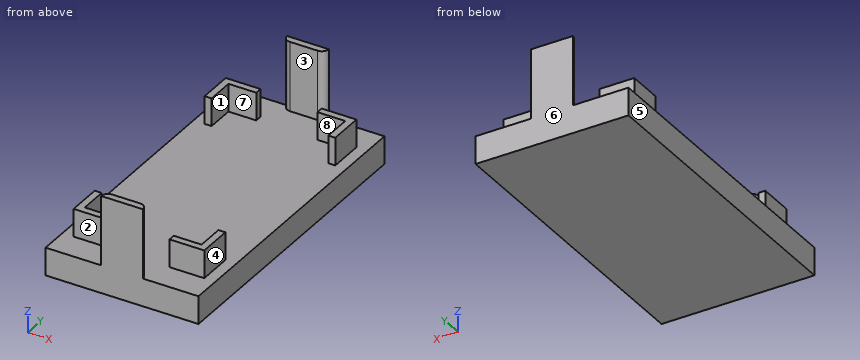
```python
from build123d import *

# Parameters (mm, degrees)
F0_W     = 110
F0_H     = 220
F1_DEPTH = 20
F3_DEPTH = 20
F4_W     = 30
F4_H     = 5
F5_DEPTH = 50
F6_R     = 4.99999


# Not quite as in the source:
# - a fillet or chamfer is up to 0.001 mm smaller than in the source, because OpenCascade refuses the exact size


with BuildPart() as f1:
    # F0 (on Top) → F1 (new body)
    with BuildSketch(Plane.XY):
        with Locations((55, -110)):
            Rectangle(F0_W, F0_H)
    extrude(amount=F1_DEPTH)

    # F2 (on face) → F3 (join)
    with BuildSketch(Plane.XY.offset(20)):
        Polygon((8, -20), (8, -45), (13, -45), (13, -25), (33, -25), (33, -20), align=None)
        Polygon((77, -20), (77, -25), (97, -25), (97, -45), (102, -45), (102, -20), align=None)
        Polygon((33, -200), (33, -195), (13, -195), (13, -175), (8, -175), (8, -200), align=None)
        Polygon((97, -175), (97, -195), (77, -195), (77, -200), (102, -200), (102, -175), align=None)
    extrude(amount=F3_DEPTH)

    # F4 (on face) → F5 (join)
    with BuildSketch(Plane.XY.offset(20)):
        with Locations((55, -2.5)):
            Rectangle(F4_W, F4_H)
        with Locations((55, -217.5)):
            Rectangle(F4_W, F4_H)
    extrude(amount=F5_DEPTH)

    # F6 (radius 5 in the source; OpenCascade refuses exactly that, so slightly less here)
    f6_edges = [f1.edges().sort_by_distance(p)[0] for p in [
        (40, -5, 45),
        (70, -5, 45),
        (40, -215, 45),
        (70, -215, 45),
    ]]
    fillet(f6_edges, radius=F6_R)


solid = f1.part
```
Here's how the part is built. I have some questions about the finished solid (model axes, mm). Face numbers are marked on the shaded views. A direction names the side the tool comes from. Round coordinates to 2 decimals unless told otherwise and drop trailing zeros. Write each loop counter-clockwise with the first axis right and the second up, starting at its lowest first coordinate (ties: lowest second). Pieces come first, ordered by that corner, then holes. Notation, with made-up numbers: M 47.5,55 L 82.5,55 A6 cw 82.5,63 Z; hole C 27,32.25 d2. An arc over 180 degrees is marked long. Answer as CSV lines item,"result". Start each with the question number.
1. Suppose I cut it at D-D on y = -141.5. Write out the boundary of the cut face in (x, z), then the cut area to 3 significant figures.
2. I'm going to push flat-ended pins straight in: pin 1 Ø3 at (x, y) = (19, -173) entering from +Z; pin 2 Ø5.5 at (y, z) = (-196.5, 25.5) entering from -X; pin 3 Ø10 at (y, z) = (-38.5, 29) entering from +X. Where does each tip first touch, or does it pass through?
3. Suppose I cut it at C-C on z = 37. Count the separate pieces of the cut face and the enclosed holes in it, then the cut area to 3 significant figures.
4. On a 3-axis mill with a long thin cutter (end or side, diameter ignored), from which of +Z, -Z, +X, -X, +Y, -Y can I reach the whole of each face in a straight line? I mean the marked faces 1, 2, 3 and 4. Say none if no direction works.
5. Thinking about a two-plate mould opening in Y: for the marked faces 5, 6, 7 and 8, which applies, released by +Y, released by -Y, zero draft, split by the parting line, or undercut?
6. I need wall thicknesses on probe 1 along Y at (x, z) = (92, 29.5); probe 2 along Y at (x, z) = (65.5, 60); probe 3 along Z at (x, y) = (38, -16.5). Which ranges of each line are inside material? Lowest first, please.
7. Suppose I cut it at B-B on y = -41. Write out the boundary of the cut face in (x, z).
Check result:
1,outline,"M 0,0 L 110,0 L 110,20 L 0,20 Z"
1,area,"2,200 mm2"
2,pin 1,"stops at z = 20"
2,pin 2,"stops at x = 8"
2,pin 3,"stops at x = 102"
3,separate pieces,"6"
3,enclosed holes,"0"
3,area,"1,180 mm2"
4,face 1,"+Z"
4,face 2,"+Z, +X, -X, -Y"
4,face 3,"+Z, +X, -X"
4,face 4,"+Z, +X, +Y, -Y"
5,face 5,"zero draft"
5,face 6,"released by +Y"
5,face 7,"undercut"
5,face 8,"undercut"
6,probe 1,"y = -200 to -195, -25 to -20"
6,probe 2,"y = -220 to -215.03, -4.97 to 0"
6,probe 3,"z = 0 to 20"
7,outline,"M 0,0 L 110,0 L 110,20 L 102,20 L 102,40 L 97,40 L 97,20 L 13,20 L 13,40 L 8,40 L 8,20 L 0,20 Z"
